```python
from build123d import *

# Parameters (mm, degrees)
CROQUIS1_W              = 3
CROQUIS1_H              = 100
CROQUIS1_W_2            = 47
CROQUIS1_H_2            = 3
SALIENTE_EXTRUIR1_DEPTH = 50
CORTAR_EXTRUIR1_DEPTH   = 100


with BuildPart() as part:
    # Croquis1 → Saliente-Extruir1 (new, symmetric)
    with BuildSketch(Plane.XY):
        Rectangle(CROQUIS1_W, CROQUIS1_H)
        with Locations((25, -48.5)):
            Rectangle(CROQUIS1_W_2, CROQUIS1_H_2)
    extrude(amount=SALIENTE_EXTRUIR1_DEPTH, both=True)

    # Croquis2 → Cortar-Extruir1 (cut)
    with BuildSketch(Plane(origin=(1.5, 0, 0), x_dir=(0, 0, -1), z_dir=(1, 0, 0))):
        Polygon((-50, 50), (50, -47), (50, 50), align=None)
    extrude(amount=-CORTAR_EXTRUIR1_DEPTH, mode=Mode.SUBTRACT)


solid = part.part
```
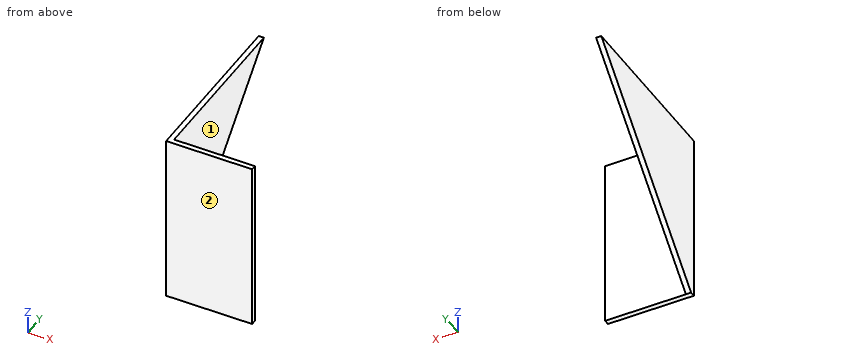
Read the model definition and answer for the solid it produces. Units are mm, in the model's axes. Face numbers are marked on the shaded views. A direction names the side the tool comes from. Coordinates: 2 decimals unless noted, no trailing zeros. Write each loop counter-clockwise with the first axis right and the second up, starting at its lowest first coordinate (ties: lowest second). Pieces come first, ordered by that corner, then holes. Notation, with made-up numbers: (-1.5, 28.25) -> (28.5, 28.25) arc R12 ccw to (28.5, 41.25) -> close; hole circle Ø1 at (40.5, -22.5). An arc over 180 degrees is marked (long way). Return JSON: item names as keys, results as strings.
1. A cutting plane is placed at A-A (z = 25). Determine the outline of the cut face in (x, y).
Found:
{"outline": "(-1.5, -50) -> (48.5, -50) -> (48.5, -47) -> (1.5, -47) -> (1.5, 25.75) -> (-1.5, 25.75) -> close"}
2. A tool of negligible diameter and unlimited length cuts with its end or side. For the marked faces 1 and 2, from which of +Z, -Z, +X, -X, +Y, -Y can it reach the whole face along a straight path? Write none if from no direction.
Found:
{"face 1": "+Z, -Z, +X, +Y", "face 2": "+Z, -Z, +X, -X, -Y"}
3. A cutting plane is placed at B-B (x = 35.5). Determine the outline of the cut face in (y, z), and give its area (3 significant figures).
Found:
{"outline": "(-50, -50) -> (-47, -50) -> (-47, 50) -> (-50, 50) -> close", "area": "300 mm2"}
4. A cutting plane is placed at C-C (z = 35). Determine the outline of the cut face in (x, y).
Found:
{"outline": "(-1.5, -50) -> (48.5, -50) -> (48.5, -47) -> (1.5, -47) -> (1.5, 35.45) -> (-1.5, 35.45) -> close"}
5. Each of these flat-tipped pins is pushed along its axis until it touches: P1, Ø5, axis at y = -14, z = -16.5, coming from the +X side; P2, Ø8, axis at x = 13.5, z = 12.5, coming from the +Y side. Where does it stop, or does it pass through?
Found:
{"P1": "x = 1.5", "P2": "y = -47"}
6. Find the intervals of material crossed by line 1 along Y through (x, z) = (44.5, -37); line 2 along X through (y, z) = (-2, 38); line 3 along Z through (x, y) = (1, 34.5), in increasing order. Write a range as from..to.
Found:
{"line 1": "-50..-47", "line 2": "-1.5..1.5", "line 3": "34.02..50"}
7. A cutting plane is placed at D-D (y = -32). Determine the outline of the cut face in (x, z), and give its area (3 significant figures).
Found:
{"outline": "(-1.5, -34.54) -> (1.5, -34.54) -> (1.5, 50) -> (-1.5, 50) -> close", "area": "254 mm2"}
